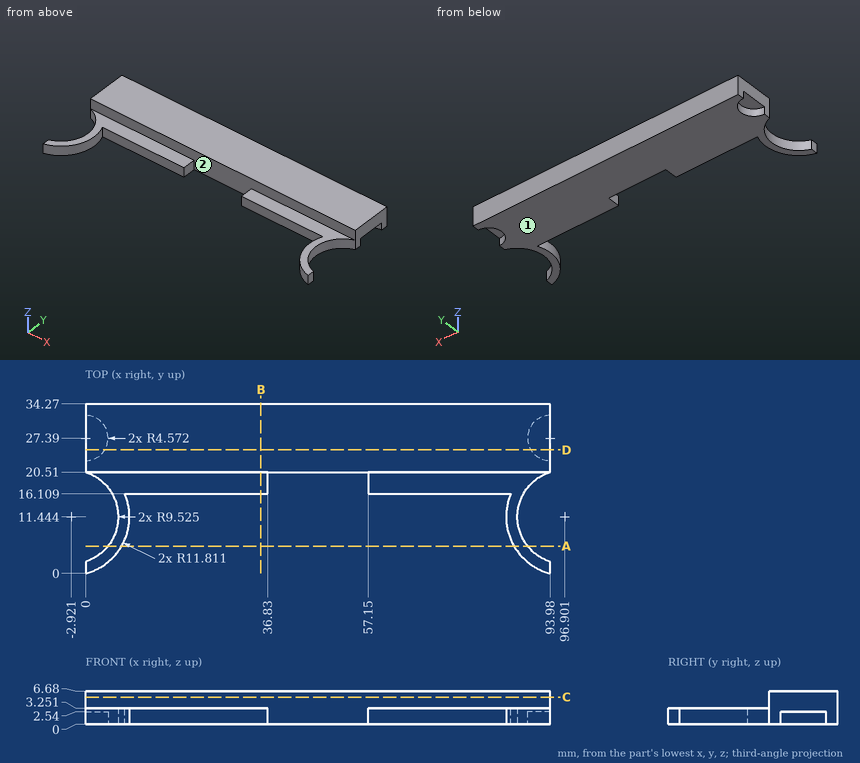
Can you work these out from the drawing? Everything is in mm from the part's minimum corner. Give positions to 0.01 mm unless a question says otherwise; leave off trailing zeros. Order: outer loops, then holes, each group sorted by start corner. A loop starts at its lowest first (then second) coordinate and runs counter-clockwise, first axis right, second up.
1. Suppose I cut it at B-B (x = 35.5). List the corners of the cut face in (y, z) for me, plus the area to 3 significant figures.
2. Suppose I cut it at D-D (y = 25). List the corners of the cut face in (x, z) for me, plus the area to 3 significant figures.
3. Suppose I cut it at A-A (y = 5.5). List the corners of the cut face in (x, z) for me (1 decimal), plus the area to 3 significant figures.
4. Suppose I cut it at C-C (z = 5.5). List the corners of the cut face in (x, y) for me.
5. Will these pins go through, and if not, where does the flat tip stop? P1, Ø1.4, axis at x = 3, y = 29, coming from the -Z side; P2, Ø6, axis at x = 13.5, y = 5.5, coming from the +Z side; P3, Ø2.5, axis at x = 74.5, z = 1.5, coming from the -Y side; P4, Ø3, axis at y = 16, z = 3, coming from the -X side.
6. We'd pull the mould along X, two halves only. Please class the marked faces 1 and 2: pulls with the +X half, pulls with the -X half, needs draft (parallel to the pull), parting line crosses it, or undercut.
7. I need wall thicknesses on L1, parallel to Y at x = 42, z = 2.25; L2, parallel to Y at x = 72.5, z = 1.5; L3, parallel to X at y = 16, z = 2.5. Which ranges of each line are inside material? Lowest first, please.
Solved:
1. outline: (16.11, 0) - (34.27, 0) - (34.27, 6.68) - (20.51, 6.68) - (20.51, 3.25) - (16.11, 3.25) - close
1. area: 106 mm2
2. outline: (0, 2.54) - (3.9, 2.54) - (3.9, 0) - (90.08, 0) - (90.08, 2.54) - (93.98, 2.54) - (93.98, 6.68) - (0, 6.68) - close
2. area: 608 mm2
3. outline: (4.5, 0) - (7.3, 0) - (7.3, 3.3) - (4.5, 3.3) - close; (86.7, 0) - (89.5, 0) - (89.5, 3.3) - (86.7, 3.3) - close
3. area: 18.0 mm2
4. outline: (0, 20.51) - (93.98, 20.51) - (93.98, 34.27) - (0, 34.27) - close
5. P1: stops at z = 2.54
5. P2: passes through
5. P3: stops at y = 16.11
5. P4: stops at x = 4.43
6. face 1: needs draft
6. face 2: undercut
7. L1: y = 20.51 to 34.27
7. L2: y = 16.11 to 34.27
7. L3: x = 5.44 to 7.98, 86 to 88.54
